from build123d import *

# Parameters (mm, degrees)
PAD_DEPTH          = 6
POCKET_DEPTH       = 2.5
POLARPATTERN_COUNT = 6


with BuildPart() as part:
    # Sketch → Pad (new body)
    with BuildSketch(Plane.XY):
        Polygon((0, 14.9), (8.602519, 14.9), (12.903779, 7.45), (12.037753, 6.95), (8.025169, 13.9), (0, 13.9), align=None)
    pad = extrude(amount=PAD_DEPTH)

    # Sketch001 → Pocket (cut)
    with BuildSketch(Plane.XY):
        Polygon((6.5, 11.25833), (11.775323, 14.304039), (6.5, 17.349749), align=None)
    pocket = extrude(amount=POCKET_DEPTH, mode=Mode.SUBTRACT)

    # PolarPattern: Pad, Pocket ×6 about axis
    polarpattern_axis = Axis((0, 0, 0), (0, 0, 1))
    for i in range(1, POLARPATTERN_COUNT):
        add(pad.rotate(polarpattern_axis, i * 360 / POLARPATTERN_COUNT))
        add(pocket.rotate(polarpattern_axis, i * 360 / POLARPATTERN_COUNT), mode=Mode.SUBTRACT)


solid = part.part
Design review of the part built by this model. Coordinates are the model's own, in mm. Coordinates: 2 decimals unless noted, no trailing zeros. Order: outer loops, then holes, each group sorted by start corner. A loop starts at its lowest first (then second) coordinate and runs counter-clockwise, first axis right, second up.
Item 1: For pin 1 Ø1 at (y, z) = (-6.5, 2) entering from +X; pin 2 Ø1.2 at (x, y) = (-8.5, 13.5) entering from -Z; pin 3 Ø3 at (y, z) = (-4.5, 3) entering from +X, all flat-tipped, find the tip position at first contact; note any pin that passes through.
Item 2: For line 1 (Y direction, x = 2, z = 2.4); line 2 (X direction, y = 11, z = 3.15); line 3 (Y direction, x = -12, z = 2.5), list the stretches that pass through material, from the lowest coordinate up.
Item 3: Take a section at C-C, the plane y = -9. Write out the cut boundary in (x, z), then the cut area to 3 significant figures.
Item 4: Take a section at B-B, the plane z = 4.35. Write out the cut boundary in (x, y), then the cut area to 3 significant figures.
Item 5: Take a section at A-A, the plane x = 5. Write out the cut boundary in (y, z), then the cut area to 3 significant figures.
Item 6: Take a section at D-D, the plane z = 2.05. Write out the cut boundary in (x, y).
Item 7: The part is to be moulded in two halves that separate along X. For faces 1 (the flat face through (-9.215, -12.826, 1.232)), 2 (the flat face through (12.5, 7.1, 0)), say which applies: pulls with the +X half, pulls with the -X half, needs draft (parallel to the pull), parting line crosses it, or undercut.
The answers:
1. pin 1: stops at x = 13.74
1. pin 2: stops at z = 2.5
1. pin 3: stops at x = 15.47
2. line 1: y = -14.9 to -13.9, 13.9 to 14.9
2. line 2: x = -10.85 to -9.7, 9.7 to 10.85
2. line 3: y = -9.02 to -7.02, 7.02 to 9.02
3. outline: (-12.01, 0) - (-10.85, 0) - (-10.85, 6) - (-12.01, 6) - close; (10.85, 0) - (12.01, 0) - (12.01, 6) - (10.85, 6) - close
3. area: 13.9 mm2
4. outline: (-17.21, 0) - (-8.6, -14.9) - (8.6, -14.9) - (17.21, 0) - (8.6, 14.9) - (-8.6, 14.9) - close; hole (-16.05, 0) - (-8.03, -13.9) - (8.03, -13.9) - (16.05, 0) - (8.03, 13.9) - (-8.03, 13.9) - close
4. area: 99.8 mm2
5. outline: (-14.9, 0) - (-13.9, 0) - (-13.9, 6) - (-14.9, 6) - close; (13.9, 0) - (14.9, 0) - (14.9, 6) - (13.9, 6) - close
5. area: 12.0 mm2
6. outline: (-16.15, -1.82) - (-9.65, -13.08) - (-8.79, -12.58) - (-15.29, -1.32) - close; (-16.15, 1.82) - (-15.29, 1.32) - (-8.79, 12.58) - (-9.65, 13.08) - close; (-6.5, -14.9) - (6.5, -14.9) - (6.5, -13.9) - (-6.5, -13.9) - close; (-6.5, 13.9) - (6.5, 13.9) - (6.5, 14.9) - (-6.5, 14.9) - close; (8.79, -12.58) - (9.65, -13.08) - (16.15, -1.82) - (15.29, -1.32) - close; (8.79, 12.58) - (15.29, 1.32) - (16.15, 1.82) - (9.65, 13.08) - close
7. face 1: undercut
7. face 2: needs draft
